```python
from build123d import *

# Parameters (mm, degrees)
BOSS_EXTRUDE1_DEPTH   = 4
BOSS_EXTRUDE1_2_DEPTH = 4
BOSS_EXTRUDE3_DEPTH   = 2
FILLET2_R             = 1
SKETCH4_W             = 14.347682942
SKETCH4_H             = 9.604544397
BOSS_EXTRUDE4_DEPTH   = 15


with BuildPart() as part:
    # Sketch1 → Boss-Extrude1 (new body)
    with BuildSketch(Plane(origin=(0, 0, 0), x_dir=(1, 0, 0), z_dir=(0, 1, 0))):
        with BuildLine():
            Line((-23.6, 10.542278437), (-17, 10.542278437))
            ThreePointArc((-17, 10.542278437), (-15.475, 9.017278437), (-17, 7.492278437))
            Line((-17, 7.492278437), (-23.6, 7.492278437))
            ThreePointArc((-23.6, 7.492278437), (-25.125, 9.017278437), (-23.6, 10.542278437))
        make_face()
    extrude(amount=BOSS_EXTRUDE1_DEPTH)



with BuildPart() as body_2:
    # Sketch1 → Boss-Extrude1 2 (new body)
    with BuildSketch(Plane(origin=(0, 0, 0), x_dir=(1, 0, 0), z_dir=(0, 1, 0))):
        with BuildLine():
            Line((23.6, 7.492278437), (17, 7.492278437))
            ThreePointArc((17, 7.492278437), (15.475, 9.017278437), (17, 10.542278437))
            Line((17, 10.542278437), (23.6, 10.542278437))
            ThreePointArc((23.6, 10.542278437), (25.125, 9.017278437), (23.6, 7.492278437))
        make_face()
    extrude(amount=BOSS_EXTRUDE1_2_DEPTH)


with BuildPart() as part_1:
    add(part.part)

    add(body_2.part)  # Boss-Extrude3 merges body 2
    # Sketch3 → Boss-Extrude3 (add)
    with BuildSketch(Plane(origin=(0, 4, 0), x_dir=(1, 0, 0), z_dir=(0, 1, 0))):
        with BuildLine():
            ThreePointArc((15.475, 9.017278437), (15.921662159, 7.938940596), (17, 7.492278437))
            Line((17, 7.492278437), (23.6, 7.492278437))
            ThreePointArc((23.6, 7.492278437), (24.678337841, 7.938940596), (25.125, 9.017278437))
            Line((25.125, 9.017278437), (25.125, 17.305889592))
            Line((25.125, 17.305889592), (25.125, 34.117278437))
            Line((25.125, 34.117278437), (-25.125, 34.117278437))
            Line((-25.125, 34.117278437), (-25.125, 17.305889592))
            Line((-25.125, 17.305889592), (-25.125, 9.017278437))
            ThreePointArc((-25.125, 9.017278437), (-24.678337841, 10.095616278), (-23.6, 10.542278437))
            Line((-23.6, 10.542278437), (-17, 10.542278437))
            ThreePointArc((-17, 10.542278437), (-15.921662159, 10.095616278), (-15.475, 9.017278437))
            Line((-15.475, 9.017278437), (-15.475, 14.117278437))
            Line((-15.475, 14.117278437), (15.475, 14.117278437))
            Line((15.475, 14.117278437), (15.475, 9.017278437))
        make_face()
        with BuildLine():
            Line((-17, 10.542278437), (-23.6, 10.542278437))
            ThreePointArc((-23.6, 10.542278437), (-25.125, 9.017278437), (-23.6, 7.492278437))
            Line((-23.6, 7.492278437), (-17, 7.492278437))
            ThreePointArc((-17, 7.492278437), (-15.475, 9.017278437), (-17, 10.542278437))
        make_face()
    extrude(amount=BOSS_EXTRUDE3_DEPTH)

    # Fillet2
    fillet2_edges = [part_1.edges().sort_by_distance(p)[0] for p in [
        (-25.125, 6, -21.567278437),
        (15.475, 6, -11.567278437),
        (-24.678337841, 6, -7.938940596),
        (-20.3, 6, -7.492278437),
        (-15.921662159, 6, -7.938940596),
        (-15.475, 6, -11.567278437),
        (15.921662159, 6, -7.938940596),
        (20.3, 6, -7.492278437),
        (24.678337841, 6, -7.938940596),
        (25.125, 6, -21.567278437),
    ]]
    fillet(fillet2_edges, radius=FILLET2_R)

    # Sketch4 → Boss-Extrude4 (add)
    with BuildSketch(Plane(origin=(0, 6, 0), x_dir=(1, 0, 0), z_dir=(0, 1, 0))):
        with Locations((-7.885296824, 29.315006239)):
            Rectangle(SKETCH4_W, SKETCH4_H)
    extrude(amount=BOSS_EXTRUDE4_DEPTH)


solid = part_1.part
```
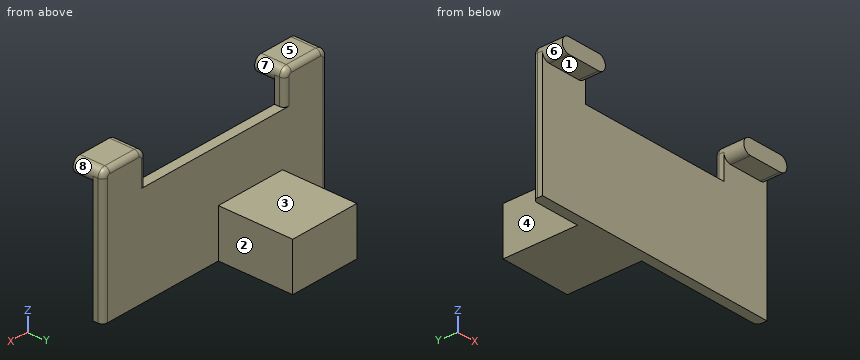
Model file for the job. Use its own axes, mm. Face numbers are marked on the shaded views. A direction names the side the tool comes from. Coordinates: 2 decimals unless noted, no trailing zeros. Loops run counter-clockwise (first coordinate to the right, second up) from the corner with the lowest first, then second, coordinate; pieces in that order, holes last. Notation, with made-up numbers: (-0.75, 81.5) -> (22.25, 81.5) arc R34 cw to (22.25, 116.5) -> close; hole circle Ø9 at (56, -4.5). An arc over 180 degrees is marked (long way). Answer as a JSON object with one key per item and string values.
Q1. Cut at A-A (y = 1.5). List the corners of the cut face in (x, z) (3 decimals).
Report:
{"outline": "(-23.6, -10.542) -> (-17, -10.542) arc R1.525 ccw to (-17, -7.492) -> (-23.6, -7.492) arc R1.525 ccw to start; (17, -10.542) -> (23.6, -10.542) arc R1.525 ccw to (23.6, -7.492) -> (17, -7.492) arc R1.525 ccw to start"}
Q2. Pull direction X, two halves, no side cores. Call the marked faces 5, 6, 7 and 8: released by +X, released by -X, zero draft, split by the parting line, or undercut.
Report:
{"face 5": "zero draft", "face 6": "released by -X", "face 7": "undercut", "face 8": "released by +X"}
Q3. 3-axis set-ups, long thin cutter, end or side, ignore diameter. For the marked faces 1, 2, 3 and 4: which of +Z, -Z, +X, -X, +Y, -Y reach the whole face in a straight line?
Report:
{"face 1": "-Z, +X, -X, -Y", "face 2": "+Z, -Z, +X, +Y", "face 3": "+Z, +X, -X, +Y", "face 4": "+Z, -Z, -X, +Y"}
Q4. Flat gauge pins, fed straight in: P1, Ø12.5, axis at x = -1.5, z = -19, coming from the -Y side; P2, Ø13, axis at x = 2.5, z = -18.5, coming from the +Y side; P3, Ø10, axis at x = 2, y = 13.5, coming from the +Z side. Where does each tip first touch, or does it go through?
Report:
{"P1": "stops at y = 4", "P2": "stops at y = 6", "P3": "stops at z = -24.51"}
Q5. Cut at D-D (y = 11.25). List the corners of the cut face in (x, z).
Report:
{"outline": "(-15.06, -34.12) -> (-0.71, -34.12) -> (-0.71, -24.51) -> (-15.06, -24.51) -> close"}
Q6. Cut at C-C (z = -32.5). List the corners of the cut face in (x, y) (3 decimals).
Report:
{"outline": "(-25.125, 4) -> (25.125, 4) -> (25.125, 5) arc R1 ccw to (24.125, 6) -> (-0.711, 6) -> (-0.711, 21) -> (-15.059, 21) -> (-15.059, 6) -> (-24.125, 6) arc R1 ccw to (-25.125, 5) -> close"}
Q7. Probe probe 1 along X at (y, z) = (14, -31); probe 2 along Y at (x, z) = (-5, -32); probe 3 along Y at (x, z) = (12, -29). List the from-to ranges inside material, lowest first.
Report:
{"probe 1": "x = -15.06 to -0.71", "probe 2": "y = 4 to 21", "probe 3": "y = 4 to 6"}
Q8. Cut at B-B (x = 21.5). List the corners of the cut face in (y, z), and give its area (3 significant figures).
Report:
{"outline": "(0, -10.54) -> (4, -10.54) -> (4, -34.12) -> (6, -34.12) -> (6, -8.49) arc R1 ccw to (5, -7.49) -> (0, -7.49) -> close", "area": "65.2 mm2"}
